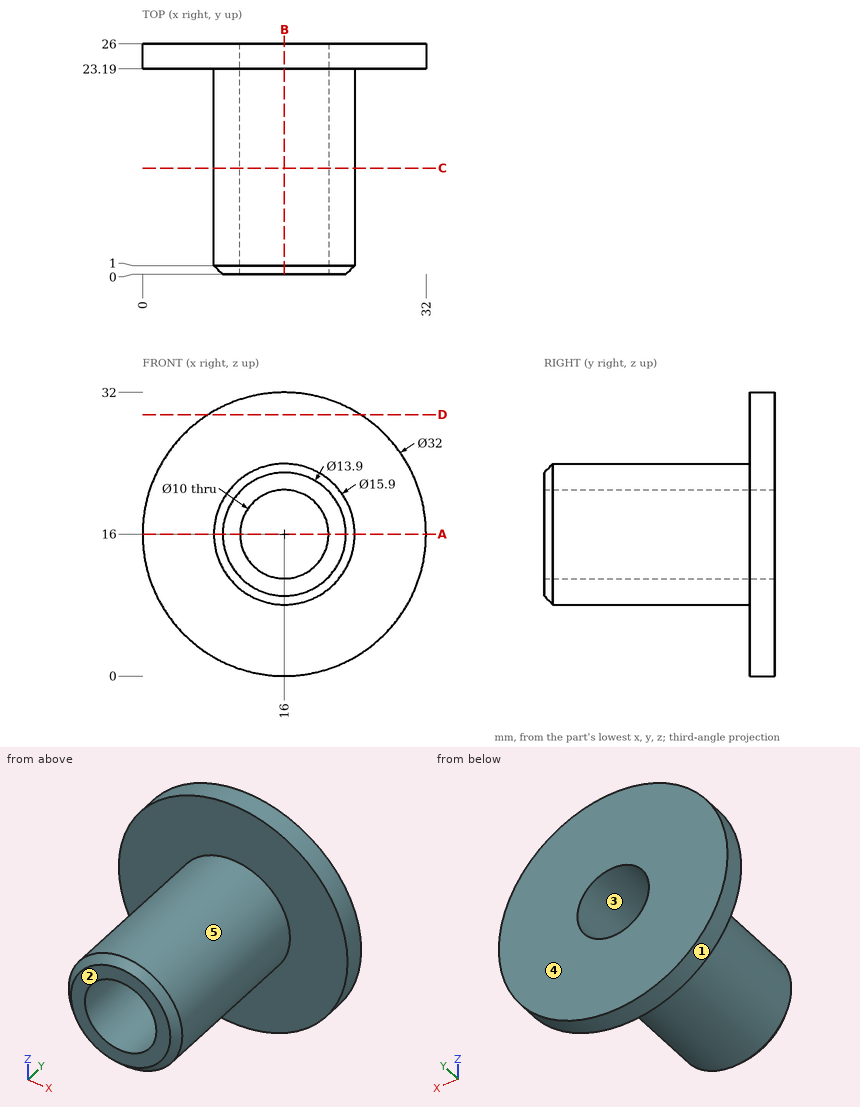
The figure shows three views and two pictorial views of one solid part (mm, origin at its lowest corner). Answer the questions. A direction names the side the tool comes from. Round coordinates to 2 decimals unless told otherwise and drop trailing zeros. Order: outer loops, then holes, each group sorted by start corner. A loop starts at its lowest first (then second) coordinate and runs counter-clockwise, first axis right, second up. Notation, with made-up numbers: M 41.25,-7.75 L 100.25,-7.75 A24 ccw 100.25,26.25 Z; hole C 6.5,-11 d9. An arc over 180 degrees is marked long. Answer in a Markdown table with one row per item. Add a question column.
1) Which of the six approach directions +Z, -Z, +X, -X, +Y, -Y give full straight-line access (tool end or side, diameter ignored) to the marked faces 4 and 5?
2) The part is cut by section D-D on z = 29.5. Determine the outline of the cut face in (x, y).
3) Consider line 1 along Z through (x, y) = (16, 14.75); line 2 along Y through (x, z) = (22.5, 22.5); line 3 along X through (y, z) = (13.25, 20). Determine where each line is inside the solid, lowest interval first. Write a range as from..to.
4) Determine the mould class of the marked faces 1, 2 and 3 for opening direction X: pulls with the +X half, pulls with the -X half, needs draft (parallel to the pull), parting line crosses it, or undercut.
5) The part is cut by section A-A on z = 16. Determine the outline of the cut face in (x, y).
6) The part is cut by section B-B on x = 16. Determine the outline of the cut face in (y, z).
7) The part is cut by section C-C on y = 12. Determine the outline of the cut face in (x, z), plus the area to 3 significant figures.
8) Flat-ended cylindrical pins translate along their axes: pin 1 Ø5 at (x, y) = (25, 10) entering from -Z; pin 2 Ø4 at (x, y) = (16, 5) entering from +Z; pin 3 Ø2 at (x, y) = (19, 5.5) entering from +Z. Find the tip coordinate at first contact, or state that the pin passes through.
Findings below:
| question | item | result |
|---|---|---|
| 1 | face 4 | +Z, -Z, +X, -X, +Y |
| 1 | face 5 | -Y |
| 2 | outline | M 7.41,23.19 L 24.59,23.19 L 24.59,26 L 7.41,26 Z |
| 3 | line 1 | z = 8.05..11, 21..23.95 |
| 3 | line 2 | y = 23.19..26 |
| 3 | line 3 | x = 9.13..13, 19..22.87 |
| 4 | face 1 | parting line crosses it |
| 4 | face 2 | needs draft |
| 4 | face 3 | undercut |
| 5 | outline | M 0,23.19 L 8.05,23.19 L 8.05,1 L 9.05,0 L 11,0 L 11,26 L 0,26 Z; M 21,0 L 22.95,0 L 23.95,1 L 23.95,23.19 L 32,23.19 L 32,26 L 21,26 Z |
| 6 | outline | M 0,9.05 L 1,8.05 L 23.19,8.05 L 23.19,0 L 26,0 L 26,11 L 0,11 Z; M 0,21 L 26,21 L 26,32 L 23.19,32 L 23.19,23.95 L 1,23.95 L 0,22.95 Z |
| 7 | outline | C 16,16 d15.9; hole C 16,16 d10 |
| 7 | area | 120 mm² |
| 8 | pin 1 | stops at z = 11.42 |
| 8 | pin 2 | stops at z = 23.95 |
| 8 | pin 3 | stops at z = 23.69 |
